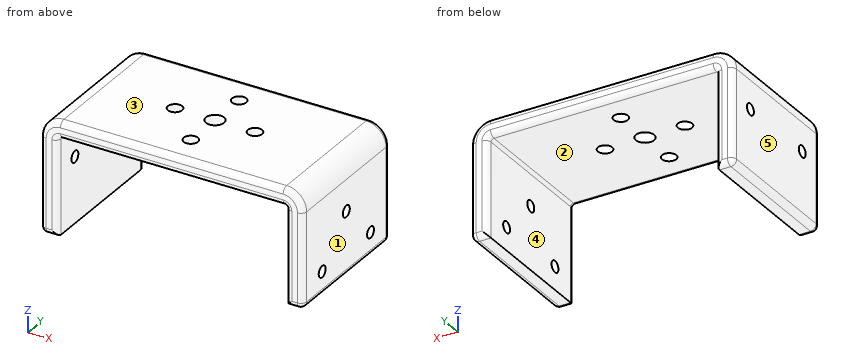
```python
from build123d import *

# Parameters (mm, degrees)
SKETCH1_W                    = 40
SKETCH1_H                    = 25
BASE_FLANGE1_DEPTH           = 3
EDGE_FLANGE1_STRIP_W         = 13
EDGE_FLANGE1_STRIP_H         = 3
EDGE_FLANGE1_STRIP_CUT_DEPTH = 25
EDGE_FLANGE1_DEPTH           = 25
EDGE_FLANGE2_STRIP_W         = 13
EDGE_FLANGE2_STRIP_H         = 3
EDGE_FLANGE2_STRIP_CUT_DEPTH = 25
EDGE_FLANGE2_DEPTH           = 25
CUT_EXTRUDE1_DEPTH           = 7
CUT_EXTRUDE2_DEPTH           = 6
FILLET1_R                    = 1
FILLET2_R                    = 1
CUT_EXTRUDE3_DEPTH           = 14


# Sheet-metal steps are written as plain solids
with BuildPart() as part:
    # Sketch1 → Base-Flange1 (new body)
    with BuildSketch(Plane.XY):
        Rectangle(SKETCH1_W, SKETCH1_H)
    extrude(amount=-BASE_FLANGE1_DEPTH)

    # Edge-Flange1 strip (across the edge) → Edge-Flange1 strip cut (cut)
    with BuildSketch(Plane(origin=(20, 12.5, -3), x_dir=(-1, 0, 0), z_dir=(0, -1, 0))):
        with Locations((-6, -1.5)):
            Rectangle(EDGE_FLANGE1_STRIP_W, EDGE_FLANGE1_STRIP_H)
    extrude(amount=EDGE_FLANGE1_STRIP_CUT_DEPTH, mode=Mode.SUBTRACT)

    # Edge-Flange1 section (across the edge) → Edge-Flange1 (add)
    with BuildSketch(Plane(origin=(20, 12.5, -3), x_dir=(-1, 0, 0), z_dir=(0, -1, 0))):
        with BuildLine():
            Line((-3, 0.5), (-3, 17))
            Line((-3, 17), (0, 17))
            Line((0, 17), (0, 0.5))
            ThreePointArc((0, 0.5), (0.146446609, 0.146446609), (0.5, 0))
            Line((0.5, 0), (0.5, -3))
            ThreePointArc((0.5, -3), (-1.974873734, -1.974873734), (-3, 0.5))
        make_face()
    extrude(amount=EDGE_FLANGE1_DEPTH)

    # Edge-Flange2 strip (across the edge) → Edge-Flange2 strip cut (cut)
    with BuildSketch(Plane(origin=(-20, -12.5, -3), x_dir=(1, 0, 0), z_dir=(0, 1, 0))):
        with Locations((-6, -1.5)):
            Rectangle(EDGE_FLANGE2_STRIP_W, EDGE_FLANGE2_STRIP_H)
    extrude(amount=EDGE_FLANGE2_STRIP_CUT_DEPTH, mode=Mode.SUBTRACT)

    # Edge-Flange2 section (across the edge) → Edge-Flange2 (add)
    with BuildSketch(Plane(origin=(-20, -12.5, -3), x_dir=(1, 0, 0), z_dir=(0, 1, 0))):
        with BuildLine():
            Line((-3, 0.5), (-3, 17))
            Line((-3, 17), (0, 17))
            Line((0, 17), (0, 0.5))
            ThreePointArc((0, 0.5), (0.146446609, 0.146446609), (0.5, 0))
            Line((0.5, 0), (0.5, -3))
            ThreePointArc((0.5, -3), (-1.974873734, -1.974873734), (-3, 0.5))
        make_face()
    extrude(amount=EDGE_FLANGE2_DEPTH)

    # Sketch12 → Cut-Extrude1 (cut)
    with BuildSketch(Plane(origin=(-20, 10.212212675, -95), x_dir=(0, -1, 0), z_dir=(-1, 0, 0))):
        with BuildLine():
            ThreePointArc((17.712212658, 87.5), (16.712212675, 86.499999984), (17.712212691, 85.5))
            ThreePointArc((17.712212691, 85.5), (18.712212675, 86.500000016), (17.712212658, 87.5))
        make_face()
        with BuildLine():
            ThreePointArc((2.712212658, 87.5), (1.712212675, 86.499999984), (2.712212691, 85.5))
            ThreePointArc((2.712212691, 85.5), (3.712212675, 86.500000016), (2.712212658, 87.5))
        make_face()
    extrude(amount=CUT_EXTRUDE1_DEPTH, mode=Mode.SUBTRACT)

    # Sketch13 → Cut-Extrude2 (cut)
    with BuildSketch(Plane(origin=(20, 10.212212675, -95), x_dir=(0, 1, 0), z_dir=(1, 0, 0))):
        with BuildLine():
            ThreePointArc((-3.21221269, 80.01), (-4.202212675, 79.019999984), (-3.212212659, 78.03))
            ThreePointArc((-3.212212659, 78.03), (-2.222212675, 79.020000016), (-3.21221269, 80.01))
        make_face()
        with BuildLine():
            ThreePointArc((-17.212212691, 80.02), (-18.212212675, 79.019999984), (-17.212212658, 78.02))
            ThreePointArc((-17.212212658, 78.02), (-16.212212675, 79.020000016), (-17.212212691, 80.02))
        make_face()
        with BuildLine():
            ThreePointArc((-10.212212691, 87.02), (-11.212212675, 86.019999984), (-10.212212658, 85.02))
            ThreePointArc((-10.212212658, 85.02), (-9.212212675, 86.020000016), (-10.212212691, 87.02))
        make_face()
    extrude(amount=CUT_EXTRUDE2_DEPTH, mode=Mode.SUBTRACT)

    # Fillet1
    fillet1_edges = [part.edges().sort_by_distance(p)[0] for p in [
        (0, 12.5, 0),
        (21.974873734, 12.5, -1.025126266),
        (21.974873734, -12.5, -1.025126266),
        (23, -12.5, -11.75),
        (23, 0, -20),
        (23, 12.5, -11.75),
        (0, -12.5, 0),
        (-21.974873734, -12.5, -1.025126266),
        (-21.974873734, 12.5, -1.025126266),
        (-23, 12.5, -11.75),
        (-23, 0, -20),
        (-23, -12.5, -11.75),
    ]]
    fillet(fillet1_edges, radius=FILLET1_R)

    # Fillet2
    # the kernel refuses this fillet: 1 mm, written as the material it takes off along each edge
    with BuildSketch(Plane(origin=(-22, 11.5, -19), x_dir=(0, 0, -1), z_dir=(0, 1, 0))) as fillet2_piece_1_section:
        Polygon((0, 0), (FILLET2_R, 0), (FILLET2_R, FILLET2_R), (0, FILLET2_R), align=None)
    fillet2_piece_1 = extrude(amount=FILLET2_R, mode=Mode.PRIVATE)
    fillet2_piece_1 = fillet2_piece_1 - Plane(origin=(-22, 11.5, -19), x_dir=(0.70710678118655, 0, 0.707106781186545), z_dir=(0, 1, 0)) * Sphere(FILLET2_R, mode=Mode.PRIVATE)
    add(fillet2_piece_1, mode=Mode.SUBTRACT)
    with BuildSketch(Plane(origin=(-22, -11.5, -19), x_dir=(0, -1, 0), z_dir=(0, 0, -1))) as fillet2_piece_2_section:
        Polygon((0, 0), (FILLET2_R, 0), (FILLET2_R, FILLET2_R), (0, FILLET2_R), align=None)
    fillet2_piece_2 = extrude(amount=FILLET2_R, mode=Mode.PRIVATE)
    fillet2_piece_2 = fillet2_piece_2 - Plane(origin=(-22, -11.5, -19), x_dir=(0.7071067811865475, 0.7071067811865477, -2.4688501310822653e-15), z_dir=(0, 0, -1)) * Sphere(FILLET2_R, mode=Mode.PRIVATE)
    add(fillet2_piece_2, mode=Mode.SUBTRACT)
    with BuildSketch(Plane(origin=(22, 11.5, -19), x_dir=(0, 0, -1), z_dir=(0, 1, 0))) as fillet2_piece_3_section:
        Polygon((0, 0), (FILLET2_R, 0), (FILLET2_R, -FILLET2_R), (0, -FILLET2_R), align=None)
    fillet2_piece_3 = extrude(amount=FILLET2_R, mode=Mode.PRIVATE)
    fillet2_piece_3 = fillet2_piece_3 - Plane(origin=(22, 11.5, -19), x_dir=(-0.70710678118655, 0, 0.707106781186545), z_dir=(0, 1, 0)) * Sphere(FILLET2_R, mode=Mode.PRIVATE)
    add(fillet2_piece_3, mode=Mode.SUBTRACT)
    with BuildSketch(Plane(origin=(22, -11.5, -19), x_dir=(0, -1, 0), z_dir=(0, 0, -1))) as fillet2_piece_4_section:
        Polygon((0, 0), (FILLET2_R, 0), (FILLET2_R, -FILLET2_R), (0, -FILLET2_R), align=None)
    fillet2_piece_4 = extrude(amount=FILLET2_R, mode=Mode.PRIVATE)
    fillet2_piece_4 = fillet2_piece_4 - Plane(origin=(22, -11.5, -19), x_dir=(-0.7071067811865475, 0.7071067811865477, -2.4688501310822653e-15), z_dir=(0, 0, -1)) * Sphere(FILLET2_R, mode=Mode.PRIVATE)
    add(fillet2_piece_4, mode=Mode.SUBTRACT)
    with BuildSketch(Plane(origin=(22, -12.5, -20), x_dir=(0, 1, 0), z_dir=(-1, 0, 0)), Plane(origin=(22, 12.5, -20), x_dir=(0, 0, 1), z_dir=(-1, 0, 0))) as fillet2_piece_5:
        with BuildLine():
            CenterArc((FILLET2_R, -FILLET2_R), FILLET2_R, 90, 90)
            Line((0, -FILLET2_R), (0, 0))
            Line((0, 0), (FILLET2_R, 0))
        make_face()
    extrude(amount=4.5, mode=Mode.SUBTRACT)
    with BuildSketch(Plane(origin=(-22, -12.5, -20), x_dir=(0, 1, 0), z_dir=(1, 0, 0)), Plane(origin=(-22, 12.5, -20), x_dir=(0, 0, 1), z_dir=(1, 0, 0))) as fillet2_piece_6:
        with BuildLine():
            CenterArc((FILLET2_R, FILLET2_R), FILLET2_R, 180, 90)
            Line((0, FILLET2_R), (0, 0))
            Line((0, 0), (FILLET2_R, 0))
        make_face()
    extrude(amount=4.5, mode=Mode.SUBTRACT)
    with BuildSketch(Plane(origin=(-19.5, 12.5, -3), x_dir=(0, 0, 1), z_dir=(1, 0, 0))) as fillet2_piece_7:
        with BuildLine():
            CenterArc((FILLET2_R, FILLET2_R), FILLET2_R, 180, 90)
            Line((0, FILLET2_R), (0, 0))
            Line((0, 0), (FILLET2_R, 0))
        make_face()
    extrude(amount=39, mode=Mode.SUBTRACT)
    with BuildSketch(Plane(origin=(19.5, 12.5, -3.5), x_dir=(1, 0, 0), z_dir=(0, 0, -1))) as fillet2_piece_8:
        with BuildLine():
            CenterArc((0.5 + FILLET2_R, FILLET2_R), FILLET2_R, 180, 90)
            Line((0.5, FILLET2_R), (0.5, 0))
            Line((0.5, 0), (0.5 + FILLET2_R, 0))
        make_face()
    revolve(axis=Axis((19.5, 12.5, -3.5), (0, -1, 0)), revolution_arc=90, mode=Mode.SUBTRACT)
    with BuildSketch(Plane(origin=(19.5, -12.5, -3.5), x_dir=(1, 0, 0), z_dir=(0, 0, -1))) as fillet2_piece_9:
        with BuildLine():
            CenterArc((0.5 + FILLET2_R, -FILLET2_R), FILLET2_R, 90, 90)
            Line((0.5 + FILLET2_R, 0), (0.5, 0))
            Line((0.5, 0), (0.5, -FILLET2_R))
        make_face()
    revolve(axis=Axis((19.5, -12.5, -3.5), (0, -1, 0)), revolution_arc=90, mode=Mode.SUBTRACT)
    with BuildSketch(Plane(origin=(20, -12.5, -22.5), x_dir=(0, 1, 0), z_dir=(0, 0, 1)), Plane(origin=(20, 12.5, -22.5), x_dir=(1, 0, 0), z_dir=(0, 0, 1))) as fillet2_piece_10:
        with BuildLine():
            CenterArc((FILLET2_R, -FILLET2_R), FILLET2_R, 90, 90)
            Line((0, -FILLET2_R), (0, 0))
            Line((0, 0), (FILLET2_R, 0))
        make_face()
    extrude(amount=19, mode=Mode.SUBTRACT)
    with BuildSketch(Plane(origin=(19.5, -12.5, -3), x_dir=(0, 1, 0), z_dir=(-1, 0, 0))) as fillet2_piece_11:
        with BuildLine():
            CenterArc((FILLET2_R, -FILLET2_R), FILLET2_R, 90, 90)
            Line((0, -FILLET2_R), (0, 0))
            Line((0, 0), (FILLET2_R, 0))
        make_face()
    extrude(amount=39, mode=Mode.SUBTRACT)
    with BuildSketch(Plane(origin=(-19.5, -12.5, -3.5), x_dir=(-1, 0, 0), z_dir=(0, 0, -1))) as fillet2_piece_12:
        with BuildLine():
            CenterArc((0.5 + FILLET2_R, FILLET2_R), FILLET2_R, 180, 90)
            Line((0.5 + FILLET2_R, 0), (0.5, 0))
            Line((0.5, 0), (0.5, FILLET2_R))
        make_face()
    revolve(axis=Axis((-19.5, -12.5, -3.5), (0, 1, 0)), revolution_arc=90, mode=Mode.SUBTRACT)
    with BuildSketch(Plane(origin=(-19.5, 12.5, -3.5), x_dir=(-1, 0, 0), z_dir=(0, 0, -1))) as fillet2_piece_13:
        with BuildLine():
            CenterArc((0.5 + FILLET2_R, -FILLET2_R), FILLET2_R, 90, 90)
            Line((0.5, -FILLET2_R), (0.5, 0))
            Line((0.5, 0), (0.5 + FILLET2_R, 0))
        make_face()
    revolve(axis=Axis((-19.5, 12.5, -3.5), (0, 1, 0)), revolution_arc=90, mode=Mode.SUBTRACT)
    with BuildSketch(Plane(origin=(-20, 12.5, -22.5), x_dir=(-1, 0, 0), z_dir=(0, 0, 1)), Plane(origin=(-20, -12.5, -22.5), x_dir=(0, 1, 0), z_dir=(0, 0, 1))) as fillet2_piece_14:
        with BuildLine():
            CenterArc((FILLET2_R, FILLET2_R), FILLET2_R, 180, 90)
            Line((0, FILLET2_R), (0, 0))
            Line((0, 0), (FILLET2_R, 0))
        make_face()
    extrude(amount=19, mode=Mode.SUBTRACT)

    # Sketch14 → Cut-Extrude3 (cut)
    with BuildSketch(Plane(origin=(1.842409503, 10.212212675, 0), x_dir=(0, 1, 0), z_dir=(0, 0, 1))):
        with BuildLine():
            ThreePointArc((-8.962212675, 8.842411376), (-10.212212675, 10.092411376), (-11.462212675, 8.842411376))
            ThreePointArc((-11.462212675, 8.842411376), (-10.212212675, 7.592411376), (-8.962212675, 8.842411376))
        make_face()
        with BuildLine():
            ThreePointArc((-3.212210801, 0.592409503), (-1.962210801, 1.842409503), (-3.212210801, 3.092409503))
            ThreePointArc((-3.212210801, 3.092409503), (-4.462210801, 1.842409503), (-3.212210801, 0.592409503))
        make_face()
        with BuildLine():
            ThreePointArc((-17.212214548, 0.592409503), (-15.962214548, 1.842409503), (-17.212214548, 3.092409503))
            ThreePointArc((-17.212214548, 3.092409503), (-18.462214548, 1.842409503), (-17.212214548, 0.592409503))
        make_face()
        with BuildLine():
            ThreePointArc((-11.462212675, -5.15759237), (-10.212212675, -6.40759237), (-8.962212675, -5.15759237))
            ThreePointArc((-8.962212675, -5.15759237), (-10.212212675, -3.90759237), (-11.462212675, -5.15759237))
        make_face()
        with BuildLine():
            ThreePointArc((-10.212212675, 0.242409503), (-8.612212675, 1.842409503), (-10.212212675, 3.442409503))
            ThreePointArc((-10.212212675, 3.442409503), (-11.812212675, 1.842409503), (-10.212212675, 0.242409503))
        make_face()
    extrude(amount=-CUT_EXTRUDE3_DEPTH, mode=Mode.SUBTRACT)


solid = part.part
```
Source: CAD feature listing. Evaluate the final solid. Frame: model axes, mm. Face numbers are marked on the shaded views. A direction names the side the tool comes from. Give positions to 0.01 mm unless a question says otherwise; leave off trailing zeros. Loops run counter-clockwise (first coordinate to the right, second up) from the corner with the lowest first, then second, coordinate; pieces in that order, holes last. Notation, with made-up numbers: (0.5, 3) - (14.5, 3) arc R18 cw to (14.5, 8) - close; hole circle Ø7 at (-15, -35). An arc over 180 degrees is marked (long way). Use CSV: the item, a comma, the result in double quotes. Start each with the question number.
1. Ray query, L1, parallel to Y at x = -21.05, z = -8.5; L2, parallel to X at y = 7.5, z = -11.75; L3, parallel to X at y = 0, z = -1.5. Return the intervals inside material, ascending.
2. Reachability of the marked faces 4 and 5 from +Z, -Z, +X, -X, +Y, -Y: full face, straight path, thin tool, end or side. Return the list, or none.
3. Section A-A (z = -10.75). Output: boundary loops of the cut face in (x, y).
4. Section B-B (y = 0). Count the separate pieces of the cut face and the enclosed holes in it, then the cut area to 3 significant figures.
5. Section D-D (y = 9.25). Output: boundary loops of the cut face in (x, z).
6. Draft query along X for the marked faces 1, 2 and 3. Return one class per face: +X half, -X half, draft (parallel to the pull), parting line (faces both ways), or undercut.
7. Section C-C (x = -14). Output: boundary loops of the cut face in (y, z).
8. Pin query (flat end, axial travel): pin 1 (2 mm diameter, centred on x = 0, y = 7, fed in from +Z); pin 2 (3 mm diameter, centred on x = 7, y = 0, fed in from -Z); pin 3 (3 mm diameter, centred on x = -7, y = 0, fed in from +Z). Return the tip coordinate at first contact, or that it passes through.
Response:
1,L1,"-12.5 to -8.5, -6.5 to 6.5, 8.5 to 12.5"
1,L2,"-23 to -20, 20 to 23"
1,L3,"-22.37 to -8.25, -5.75 to -1.6, 1.6 to 5.75, 8.25 to 22.37"
2,face 4,"-Z, +Y, -Y"
2,face 5,"+Z, -Z, -X, +Y, -Y"
3,outline,"(-23, -11.5) arc R1 ccw to (-22, -12.5) - (-21, -12.5) arc R1 ccw to (-20, -11.5) - (-20, 11.5) arc R1 ccw to (-21, 12.5) - (-22, 12.5) arc R1 ccw to (-23, 11.5) - close; (20, -11.5) arc R1 ccw to (21, -12.5) - (22, -12.5) arc R1 ccw to (23, -11.5) - (23, 11.5) arc R1 ccw to (22, 12.5) - (21, 12.5) arc R1 ccw to (20, 11.5) - close"
4,separate pieces,"5"
4,enclosed holes,"0"
4,area,"204 mm²"
5,outline,"(-23, -19) arc R1 ccw to (-22, -20) - (-20, -20) - (-20, -3.5) arc R0.5 cw to (-19.5, -3) - (19.5, -3) arc R0.5 cw to (20, -3.5) - (20, -20) - (22, -20) arc R1 ccw to (23, -19) - (23, -3.5) arc R3.5 ccw to (19.5, 0) - (-19.5, 0) arc R3.5 ccw to (-23, -3.5) - close"
6,face 1,"+X half"
6,face 2,"undercut"
6,face 3,"draft"
7,outline,"(-12.5, -2) arc R1 ccw to (-11.5, -3) - (11.5, -3) arc R1 ccw to (12.5, -2) - (12.5, -1) arc R1 ccw to (11.5, 0) - (-11.5, 0) arc R1 ccw to (-12.5, -1) - close"
8,pin 1,"through"
8,pin 2,"z = -3"
8,pin 3,"z = 0"
